Design review of the part built by this model. Coordinates are the model's own, in mm. A direction names the side the tool comes from. Give positions to 0.01 mm unless a question says otherwise; leave off trailing zeros. Loops run counter-clockwise (first coordinate to the right, second up) from the corner with the lowest first, then second, coordinate; pieces in that order, holes last. Notation, with made-up numbers: M -21,65 L -13,65 A13 cw -13,71 Z; hole C -13.5,73 d1. An arc over 180 degrees is marked long. Answer as CSV lines item,"result".
```python
from build123d import *

# Parameters (mm, degrees)
SKETCH1_R                       = 36.3855
BOSS_EXTRUDE1_DEPTH             = 6.35
TAP_DRILL_FOR_M3X0_5_TAP2_D     = 2.5
TAP_DRILL_FOR_M3X0_5_TAP2_DEPTH = 3.175
TAP_DRILL_FOR_M3X0_5_TAP2_TIP   = 0.751075774
SKETCH7_R                       = 8.001
CUT_EXTRUDE1_DEPTH              = 52.847195879


with BuildPart() as part:
    # Sketch1 → Boss-Extrude1 (new body)
    with BuildSketch(Plane(origin=(0, 0, 0), x_dir=(1, 0, 0), z_dir=(0, 1, 0))):
        with Locations(Location((0, 0, 0), (0, 0, 270))):
            Circle(SKETCH1_R)
    extrude(amount=BOSS_EXTRUDE1_DEPTH)

    # Tap Drill for M3x0.5 Tap2
    with Locations(Plane(origin=(0, 6.35, 0), x_dir=(1, 0, 0), z_dir=(0, 1, 0))):
        with Locations((0, 17.78), (0, -17.78)):
            Hole(TAP_DRILL_FOR_M3X0_5_TAP2_D / 2, depth=TAP_DRILL_FOR_M3X0_5_TAP2_DEPTH)
            with Locations((0, 0, -(TAP_DRILL_FOR_M3X0_5_TAP2_DEPTH + TAP_DRILL_FOR_M3X0_5_TAP2_TIP / 2))):  # 118° drill point
                Cone(0, TAP_DRILL_FOR_M3X0_5_TAP2_D / 2, TAP_DRILL_FOR_M3X0_5_TAP2_TIP, mode=Mode.SUBTRACT)

    # Sketch7 → Cut-Extrude1 (cut, through all)
    with BuildSketch(Plane(origin=(0, 6.35, 0), x_dir=(1, 0, 0), z_dir=(0, 1, 0))):
        with Locations(Location((0, 0, 0), (0, 0, 270))):
            Circle(SKETCH7_R)
    extrude(amount=-CUT_EXTRUDE1_DEPTH, mode=Mode.SUBTRACT)


solid = part.part
```
1. For P1, Ø1.5, axis at x = 0, z = -17.78, coming from the -Y side; P2, Ø1.5, axis at x = 0, z = 17.78, coming from the +Y side; P3, Ø1, axis at x = 4.5, y = 5.5, coming from the -Z side, all flat-tipped, find the tip position at first contact; note any pin that passes through.
Answer block:
P1,"y = 0"
P2,"y = 2.87"
P3,"z = -36.16"
2. The part is to be moulded in two halves that separate along X. For faces 3 (the flat face through (9, 0, -1)), 4 (the cylindrical face through (2.403, 3.219, 7.632)), 5 (the cylindrical face through (-35.52, 3.13, -7.89)), say which applies: pulls with the +X half, pulls with the -X half, needs draft (parallel to the pull), parting line crosses it, or undercut.
Answer block:
face 3,"needs draft"
face 4,"undercut"
face 5,"parting line crosses it"
3. We need section A-A, the plane z = 0. Write out the cut boundary in (x, y).
Answer block:
outline,"M -36.39,0 L -8,0 L -8,6.35 L -36.39,6.35 Z; M 8,0 L 36.39,0 L 36.39,6.35 L 8,6.35 Z"
4. For faces 1 (the flat face through (9, 6.35, -1)), 2 (the cylindrical face through (0.27, 4.74, -16.56)), list the 3-axis set-ups (+Z, -Z, +X, -X, +Y, -Y) from which the entire face can be reached by the end or side of a thin tool; tool diameter is ignored.
Answer block:
face 1,"+Z, -Z, +X, -X, +Y"
face 2,"+Y"
5. We need section C-C, the plane x = -6.5. Write out the cut boundary in (y, z), plus the area to 3 significant figures.
Answer block:
outline,"M 0,-35.8 L 6.35,-35.8 L 6.35,-4.67 L 0,-4.67 Z; M 0,4.67 L 6.35,4.67 L 6.35,35.8 L 0,35.8 Z"
area,"395 mm²"
6. We need section D-D, the plane y = 1.5. Write out the cut boundary in (x, z), plus the area to 3 significant figures.
Answer block:
outline,"C 0,0 d72.77; hole C 0,0 d16"
area,"3,960 mm²"
7. To check wall thickness, follow L1, parallel to X at y = 4.5, z = 0; L2, parallel to X at y = 2.75, z = -4; L3, parallel to Z at x = 3, y = 5.5. State the ranges of each line that lie inside material, in increasing order. Write a range as [from, to].
Answer block:
L1,"[-36.39, -8], [8, 36.39]"
L2,"[-36.16, -6.93], [6.93, 36.16]"
L3,"[-36.26, -7.42], [7.42, 36.26]"
8. We need section B-B, the plane y = 5.25. Write out the cut boundary in (x, z).
Answer block:
outline,"C 0,0 d72.77; hole C 0,0 d16; hole C 0,-17.78 d2.5; hole C 0,17.78 d2.5"
